Source: CAD feature listing. Evaluate the final solid. Frame: model axes, mm. A direction names the side the tool comes from. Coordinates: 2 decimals unless noted, no trailing zeros. Order: outer loops, then holes, each group sorted by start corner. A loop starts at its lowest first (then second) coordinate and runs counter-clockwise, first axis right, second up. Notation, with made-up numbers: (24, 80) -> (63, 80) arc R17 cw to (63, 95) -> close; hole circle Ø6 at (85, 9). An arc over 180 degrees is marked (long way). Write item = value, one per line. Start each with the question number.
Item 1: Mould query, pull axis X, two halves, no side actions, for faces 4 (the flat face through (41, 0, -1)), 5 (the flat face through (82.55, 3, 1)), 6 (the cylindrical face through (77.303, 1.609, -74.997)). Classes: released by +X, released by -X, zero draft, split by the parting line, or undercut.
Item 2: Section query B-B (x = 10). Output: boundary loops of the cut face in (y, z).
Item 3: Set-up query: faces 1 (the flat face through (76, 2.235, 78)), 2 (the flat face through (41, 3, 32.4)), 3 (the flat face through (40, 3, 82.55)). Return all of +Z, -Z, +X, -X, +Y, -Y with unobstructed straight access to the full face (end or side cutting, diameter ignored); none if empty.
Item 4: Section query A-A (z = 50.5). Output: boundary loops of the cut face in (x, y) (3 decimals), then the cut area to 3 significant figures.
Item 5: Ray query, line 1 along Z through (x, y) = (43.5, 1); line 2 along X through (y, z) = (1.25, 38.5) (3 decimals); line 3 along X through (y, z) = (3, 48) (3 decimals). Return the intervals inside material, ascending. Write a range as [from, to].
Item 6: Contact query for flat-ended pins moving along their axis: pin 1 (3 mm diameter, centred on x = 76.2, z = -76.2, fed in from +Y); pin 2 (0.8 mm diameter, centred on y = 0.5, z = -74.5, fed in from +X); pin 3 (4 mm diameter, centred on x = 76.2, z = 76.2, fed in from -Y). Output: stop coordinate, or through.
```python
from build123d import *

# Parameters (mm, degrees)
BOSS_EXTRUDE1_DEPTH                            = 6.35
LPATTERN1_COUNT                                = 6
LPATTERN1_PITCH                                = 25.4
LPATTERN2_COUNT                                = 3
LPATTERN2_PITCH                                = 25.4
SKETCH5_W                                      = 50.8
SKETCH5_H                                      = 38.1
FEEDTHROUGHS_DEPTH                             = 6.35
F_4_40_TAPPED_HOLE_Y_D                         = 2.2606
FILLET1_R                                      = 1
CBORE_FOR_4_SOCKET_HEAD_CAP_SCREW1_D           = 3.2639
CBORE_FOR_4_SOCKET_HEAD_CAP_SCREW1_DEPTH       = 8.89
CBORE_FOR_4_SOCKET_HEAD_CAP_SCREW1_CBORE_D     = 8.509
CBORE_FOR_4_SOCKET_HEAD_CAP_SCREW1_CBORE_DEPTH = 4.1148
CBORE_FOR_4_SOCKET_HEAD_CAP_SCREW1_TIP         = 0.980574487
F_8_32_TAPPED_HEAT_STRAP_D                     = 3.4544
F_4_40_TAPPED_GRID_D                           = 2.2606
LPATTERN4_COUNT                                = 6
LPATTERN4_PITCH                                = 12.7
LPATTERN4_COUNT_DIR2                           = 3
LPATTERN4_PITCH_DIR2                           = 12.7
LPATTERN5_COUNT                                = 2
LPATTERN5_PITCH                                = 12.7
LPATTERN5_COUNT_DIR2                           = 5
LPATTERN5_PITCH_DIR2                           = 12.7
BAR_CUTOUTS_R                                  = 1
BAR_CUTOUTS_W                                  = 12.7
BAR_CUTOUTS_H                                  = 12.7
CUT_EXTRUDE1_DEPTH                             = 1
FILLET2_R                                      = 1


with BuildPart() as part:
    # Sketch1 → Boss-Extrude1 (new body)
    with BuildSketch(Plane(origin=(0, 0, 0), x_dir=(1, 0, 0), z_dir=(0, 1, 0))):
        with BuildLine():
            Line((0, -15), (0, -82.55))
            Line((0, -82.55), (82.55, -82.55))
            Line((82.55, -82.55), (82.55, 82.55))
            Line((82.55, 82.55), (0, 82.55))
            Line((0, 82.55), (0, 15))
            ThreePointArc((0, 15), (15, 0), (0, -15))
        make_face()
    extrude(amount=BOSS_EXTRUDE1_DEPTH)

    # Sketch2 → #4-40 Tapped Hole - Z (revolve, cut)
    with BuildSketch(Plane(origin=(82.55, 3.175, 63.5), x_dir=(0, 0, -1), z_dir=(0, 1, 0))):
        Polygon((0, 0), (0, 8.279152758), (1.1303, 7.6), (1.1303, 0), align=None)
    f_4_40_tapped_hole_z = revolve(axis=Axis((88.9, 3.175, 63.5), (-1, 0, 0)), mode=Mode.SUBTRACT)

    # LPattern1: #4-40 Tapped Hole - Z ×6
    with Locations(*[(0, 0, -i * LPATTERN1_PITCH) for i in range(1, LPATTERN1_COUNT)]):
        add(f_4_40_tapped_hole_z, mode=Mode.SUBTRACT)

    # Sketch3 → #4-40 Tapped Hole - X (revolve, cut)
    with BuildSketch(Plane(origin=(63.5, 3.175, 82.55), x_dir=(0, -1, 0), z_dir=(1, 0, 0))):
        Polygon((0, 0), (0, 8.279152758), (1.1303, 7.6), (1.1303, 0), align=None)
    f_4_40_tapped_hole_x = revolve(axis=Axis((63.5, 3.175, 88.9), (0, 0, -1)), mode=Mode.SUBTRACT)

    # LPattern2: #4-40 Tapped Hole - X ×3
    with Locations(*[(-i * LPATTERN2_PITCH, 0, 0) for i in range(1, LPATTERN2_COUNT)]):
        add(f_4_40_tapped_hole_x, mode=Mode.SUBTRACT)

    # Mirror1: #4-40 Tapped Hole - X across plane
    add(f_4_40_tapped_hole_x.mirror(Plane.XY), mode=Mode.SUBTRACT)

    # Mirror1 copy 1 sketch → Mirror1 copy 1 (revolve, cut)
    with BuildSketch(Plane(origin=(38.1, 3.175, -82.55), x_dir=(0, -1, 0), z_dir=(1, 0, 0))):
        Polygon((0, 0), (0, -8.279152758), (1.1303, -7.6), (1.1303, 0), align=None)
    revolve(axis=Axis((38.1, 3.175, -88.9), (0, 0, -1)), mode=Mode.SUBTRACT)

    # Mirror1 copy 2 sketch → Mirror1 copy 2 (revolve, cut)
    with BuildSketch(Plane(origin=(12.7, 3.175, -82.55), x_dir=(0, -1, 0), z_dir=(1, 0, 0))):
        Polygon((0, 0), (0, -8.279152758), (1.1303, -7.6), (1.1303, 0), align=None)
    revolve(axis=Axis((12.7, 3.175, -88.9), (0, 0, -1)), mode=Mode.SUBTRACT)

    # Sketch5 → Feedthroughs (cut)
    with BuildSketch(Plane(origin=(0, 0, 0), x_dir=(1, 0, 0), z_dir=(0, 1, 0))):
        with Locations((41.275, 51.45)):
            Rectangle(SKETCH5_W, SKETCH5_H)
        with Locations((41.275, -51.45)):
            Rectangle(SKETCH5_W, SKETCH5_H)
    extrude(amount=FEEDTHROUGHS_DEPTH, mode=Mode.SUBTRACT)

    # #4-40 Tapped Hole - Y (through all)
    with Locations(Plane(origin=(53.975, 6.35, -73.675), x_dir=(0, 0, 1), z_dir=(0, 1, 0))):
        with Locations((0, 0), (9.525, 15.875), (44.45, 0), (44.45, -25.4), (9.525, -41.275), (0, -25.4), (34.925, -41.275), (34.925, 15.875)):
            f_4_40_tapped_hole_y = Hole(F_4_40_TAPPED_HOLE_Y_D / 2)

    # #4-40 Tapped Hole - Y Mirror: #4-40 Tapped Hole - Y across plane
    add(f_4_40_tapped_hole_y.mirror(Plane.XY), mode=Mode.SUBTRACT)

    # Fillet1
    fillet1_edges = [part.edges().sort_by_distance(p)[0] for p in [
        (15.875, 3.175, -70.5),
        (15.875, 3.175, -32.4),
        (66.675, 3.175, -32.4),
        (66.675, 3.175, -70.5),
        (15.875, 3.175, 70.5),
        (66.675, 3.175, 70.5),
        (66.675, 3.175, 32.4),
        (15.875, 3.175, 32.4),
    ]]
    fillet(fillet1_edges, radius=FILLET1_R)

    # CBORE for #4 Socket Head Cap Screw1
    with Locations(Plane(origin=(76.2, 6.35, -76.2), x_dir=(0, 0, 1), z_dir=(0, 1, 0))):
        with Locations((0, 0), (152.4, 0)):
            CounterBoreHole(CBORE_FOR_4_SOCKET_HEAD_CAP_SCREW1_D / 2, CBORE_FOR_4_SOCKET_HEAD_CAP_SCREW1_CBORE_D / 2, CBORE_FOR_4_SOCKET_HEAD_CAP_SCREW1_CBORE_DEPTH, depth=CBORE_FOR_4_SOCKET_HEAD_CAP_SCREW1_DEPTH)
            with Locations((0, 0, -(CBORE_FOR_4_SOCKET_HEAD_CAP_SCREW1_DEPTH + CBORE_FOR_4_SOCKET_HEAD_CAP_SCREW1_TIP / 2))):  # 118° drill point
                Cone(0, CBORE_FOR_4_SOCKET_HEAD_CAP_SCREW1_D / 2, CBORE_FOR_4_SOCKET_HEAD_CAP_SCREW1_TIP, mode=Mode.SUBTRACT)

    # #8-32 Tapped Heat strap (through all)
    with Locations(Plane(origin=(26.35, 6.35, -6.35), x_dir=(0, 0, 1), z_dir=(0, 1, 0))):
        with Locations((0, 0), (0, 12.7), (0, 25.4), (0, 38.1), (12.7, 38.1), (12.7, 25.4), (12.7, 12.7), (12.7, 0)):
            Hole(F_8_32_TAPPED_HEAT_STRAP_D / 2)

    # #4-40 Tapped Grid (through all)
    with Locations(Plane(origin=(70.7, 6.35, -6.35), x_dir=(0, 0, 1), z_dir=(0, 1, 0))):
        with Locations((0, 0)):
            f_4_40_tapped_grid = Hole(F_4_40_TAPPED_GRID_D / 2)

    # LPattern4: 4-40 Tapped Grid 6 × 3, 3 skipped
    with Locations(*[(-i * LPATTERN4_PITCH, 0, j * LPATTERN4_PITCH_DIR2) for i in range(LPATTERN4_COUNT) for j in range(LPATTERN4_COUNT_DIR2) if (i, j) not in ((0, 0), (5, 0), (5, 1), (5, 2))]):
        add(f_4_40_tapped_grid, mode=Mode.SUBTRACT)

    # LPattern5: 4-40 Tapped Grid 2 × 5, 4 skipped
    with Locations(*[(-j * LPATTERN5_PITCH_DIR2, 0, -i * LPATTERN5_PITCH) for i in range(LPATTERN5_COUNT) for j in range(LPATTERN5_COUNT_DIR2) if (i, j) not in ((0, 0), (0, 1), (0, 2), (0, 3), (0, 4))]):
        add(f_4_40_tapped_grid, mode=Mode.SUBTRACT)

    # Bar_cutouts → Cut-Extrude1 (cut)
    with BuildSketch(Plane(origin=(0, 0, 0), x_dir=(1, 0, 0), z_dir=(0, 1, 0))):
        with Locations((69.85, 69.85)):
            Circle(BAR_CUTOUTS_R)
        with Locations((76.2, 76.2)):
            Rectangle(BAR_CUTOUTS_W, BAR_CUTOUTS_H)
        with BuildLine():
            ThreePointArc((70.85, 69.85), (70.557106781, 70.557106781), (69.85, 70.85))
            Line((69.85, 70.85), (69.85, 69.85))
            Line((69.85, 69.85), (70.85, 69.85))
        make_face()
        with BuildLine():
            Line((69.85, 69.85), (69.85, 70.85))
            ThreePointArc((69.85, 70.85), (69.142893219, 69.142893219), (70.85, 69.85))
            Line((70.85, 69.85), (69.85, 69.85))
        make_face()
        with BuildLine():
            ThreePointArc((69.85, -70.85), (70.557106781, -70.557106781), (70.85, -69.85))
            Line((70.85, -69.85), (69.85, -69.85))
            Line((69.85, -69.85), (69.85, -70.85))
        make_face()
        with BuildLine():
            Line((69.85, -69.85), (70.85, -69.85))
            ThreePointArc((70.85, -69.85), (69.142893219, -69.142893219), (69.85, -70.85))
            Line((69.85, -70.85), (69.85, -69.85))
        make_face()
        with Locations((69.85, -69.85)):
            Circle(BAR_CUTOUTS_R)
        with Locations((76.2, -76.2)):
            Rectangle(BAR_CUTOUTS_W, BAR_CUTOUTS_H)
    extrude(amount=CUT_EXTRUDE1_DEPTH, mode=Mode.SUBTRACT)

    # Fillet2
    fillet2_edges = [part.edges().sort_by_distance(p)[0] for p in [
        (82.55, 3.675, -82.55),
        (82.55, 3.675, 82.55),
    ]]
    fillet(fillet2_edges, radius=FILLET2_R)


solid = part.part
```
Computed:
q1.face_4 = zero draft
q1.face_5 = released by +X
q1.face_6 = undercut
q2.outline = (0, -82.55) -> (6.35, -82.55) -> (6.35, -11.18) -> (0, -11.18) -> close; (0, 11.18) -> (6.35, 11.18) -> (6.35, 82.55) -> (0, 82.55) -> close
q3.face_1 = +Y
q3.face_2 = +Y, -Y
q3.face_3 = +Z, +X, -X, +Y, -Y
q4.outline = (0, 0) -> (15.875, 0) -> (15.875, 6.35) -> (0, 6.35) -> close; (66.675, 0) -> (82.55, 0) -> (82.55, 6.35) -> (66.675, 6.35) -> close
q4.area = 202 mm^2
q5.line_1 = [-82.55, -70.5], [-32.4, 32.4], [70.5, 82.55]
q5.line_2 = [0, 11.598], [13.802, 15.875], [66.675, 68.748], [70.952, 82.55]
q5.line_3 = [0, 15.875], [66.675, 82.55]
q6.pin_1 = through
q6.pin_2 = 69.85
q6.pin_3 = 1
